from build123d import *

# Parameters (mm, degrees)
SKETCH_W        = 68
SKETCH_H        = 44
SKETCH_R        = 1.75
SKETCH_R_2      = 1.2
PAD_DEPTH       = 5
SKETCH001_R     = 3.6
SKETCH001_R_2   = 2.65
POCKET_DEPTH    = 2.5
SKETCH002_W     = 1.5
SKETCH002_H     = 4
PAD001_DEPTH    = 2
SKETCH003_R     = 0.9
POCKET001_DEPTH = 5
SKETCH004_W     = 16
SKETCH004_H     = 17
POCKET002_DEPTH = 1
SKETCH005_W     = 8
SKETCH005_H     = 3
PAD002_DEPTH    = 1
POCKET003_DEPTH = 27


with BuildPart() as part:
    # Sketch → Pad (new body)
    with BuildSketch(Plane.XY):
        Rectangle(SKETCH_W, SKETCH_H)
        with Locations((18, -16.75)):
            Circle(SKETCH_R, mode=Mode.SUBTRACT)
        with Locations((-18, -16.75)):
            Circle(SKETCH_R, mode=Mode.SUBTRACT)
        with Locations((-25, 14)):
            Circle(SKETCH_R_2, mode=Mode.SUBTRACT)
    extrude(amount=PAD_DEPTH)

    # Sketch001 (on Face9 of Pad) → Pocket (cut)
    with BuildSketch(Plane.XY.offset(5)):
        with Locations((-18, -16.75)):
            Circle(SKETCH001_R)
        with Locations((18, -16.75)):
            Circle(SKETCH001_R)
        with Locations((-25, 14)):
            Circle(SKETCH001_R_2)
    extrude(amount=-POCKET_DEPTH, mode=Mode.SUBTRACT)

    # Sketch002 (on Face5 of Pocket) → Pad001 (join)
    with BuildSketch(Plane.XY.offset(5)):
        Polygon((-16.5, -21), (16.5, -21), (16.5, -20.35), (18, -20.35), (18, -22), (-18, -22), (-18, -20.35), (-16.5, -20.35), align=None)
        Polygon((16.5, 15.4), (16.5, 13.4), (18, 13.4), (18, 22), (-18, 22), (-18, 13.4), (-16.5, 13.4), (-16.5, 15.4), align=None)
        with Locations((-17.25, -2.8)):
            Rectangle(SKETCH002_W, SKETCH002_H)
        with Locations((17.25, -2.8)):
            Rectangle(SKETCH002_W, SKETCH002_H)
    extrude(amount=PAD001_DEPTH)

    # Sketch003 (on Face34 of Pad001) → Pocket001 (cut)
    with BuildSketch(Plane.XY.offset(7)):
        with Locations((0, 16.5)):
            Circle(SKETCH003_R)
    extrude(amount=-POCKET001_DEPTH, mode=Mode.SUBTRACT)

    # Sketch004 (on Face5 of Pocket001) → Pocket002 (cut)
    with BuildSketch(Plane.XY.offset(5)):
        with Locations((26, 6.3)):
            Rectangle(SKETCH004_W, SKETCH004_H)
        with Locations((26, -11.9)):
            Rectangle(SKETCH004_W, SKETCH004_H)
        with Locations((-26, 6.3)):
            Rectangle(SKETCH004_W, SKETCH004_H)
        with Locations((-26, -11.9)):
            Rectangle(SKETCH004_W, SKETCH004_H)
    extrude(amount=-POCKET002_DEPTH, mode=Mode.SUBTRACT)

    # Sketch005 (on Face21 of Pocket002) → Pad002 (join, symmetric)
    with BuildSketch(Plane.XY.offset(7)):
        with Locations((-9.5, -20.5)):
            Rectangle(SKETCH005_W, SKETCH005_H)
        with Locations((9.5, -20.5)):
            Rectangle(SKETCH005_W, SKETCH005_H)
    extrude(amount=PAD002_DEPTH, both=True)

    # Sketch006 (on Face62 of Pad002) → Pocket003 (cut)
    with BuildSketch(Plane.YZ.offset(13.5)):
        Polygon((-19, 6), (-21, 6), (-19, 8), align=None)
    extrude(amount=-POCKET003_DEPTH, mode=Mode.SUBTRACT)


solid = part.part
Read the model definition and answer for the solid it produces. Units are mm, in the model's axes. A direction names the side the tool comes from. Round coordinates to 2 decimals unless told otherwise and drop trailing zeros. Write each loop counter-clockwise with the first axis right and the second up, starting at its lowest first coordinate (ties: lowest second). Pieces come first, ordered by that corner, then holes.
Q1. Find section A-A on x = -25. Determine the outline of the cut face in (y, z), and give its area (3 significant figures).
Values:
outline: (-22, 0) - (12.8, 0) - (12.8, 2.5) - (11.35, 2.5) - (11.35, 4) - (-2.2, 4) - (-2.2, 5) - (-3.4, 5) - (-3.4, 4) - (-20.4, 4) - (-20.4, 5) - (-22, 5) - close; (15.2, 0) - (22, 0) - (22, 5) - (16.65, 5) - (16.65, 2.5) - (15.2, 2.5) - close
area: 170 mm2
Q2. Flat-ended cylindrical pins translate along their axes: P1, Ø0.6, axis at y = -2, z = 6, coming from the +X side; P2, Ø12, axis at x = 13.5, y = 17.5, coming from the +Z side; P3, Ø2, axis at x = -17.5, y = -15.5, coming from the +Z side. Find the tip coordinate at first contact, or state that the pin passes through.
Values:
P1: stops at x = 18
P2: stops at z = 7
P3: stops at z = 2.5
Q3. The mould has two halves that part along Y. Classify faces 4 (the face through (0, 22, 3)), 5 (the face through (26, -12, 4)), 6 (the face through (-26, -12, 4)), 7 (the face through (-16.2, -21.3, 7)): released by +Y, released by -Y, zero draft, split by the parting line, or undercut.
Values:
face 4: released by +Y
face 5: undercut
face 6: undercut
face 7: zero draft
Q4. Find section B-B on y = -16.75. Determine the outline of the cut face in (x, z).
Values:
outline: (-34, 0) - (-19.75, 0) - (-19.75, 2.5) - (-21.6, 2.5) - (-21.6, 4) - (-34, 4) - close; (-16.25, 0) - (16.25, 0) - (16.25, 2.5) - (14.4, 2.5) - (14.4, 5) - (-14.4, 5) - (-14.4, 2.5) - (-16.25, 2.5) - close; (19.75, 0) - (34, 0) - (34, 4) - (21.6, 4) - (21.6, 2.5) - (19.75, 2.5) - close
Q5. Find section D-D on y = -6.5. Determine the outline of the cut face in (x, z), and give its area (3 significant figures).
Values:
outline: (-34, 0) - (34, 0) - (34, 4) - (18, 4) - (18, 5) - (-18, 5) - (-18, 4) - (-34, 4) - close
area: 308 mm2
Q6. Find section C-C on x = -9. Determine the outline of the cut face in (y, z), and give its area (3 significant figures).
Values:
outline: (-22, 0) - (22, 0) - (22, 7) - (15.4, 7) - (15.4, 5) - (-21, 5) - (-21, 6) - (-19, 8) - (-22, 8) - close
area: 238 mm2
Q7. Straight lines are drawn through the part: line 1 (Y direction, x = 18, z = 3.95); line 2 (X direction, y = -14, z = 3.5); line 3 (Z direction, x = 21.5, y = 1.5). For each, find the intervals that lie inside material, in ascending order.
Values:
line 1: y = -22 to -20.35, -13.15 to 22
line 2: x = -34 to -20.32, -15.68 to 15.68, 20.32 to 34
line 3: z = 0 to 4
Q8. A tool of negligible diameter and unlimited length cuts with its end or side. For faces 1 (the face through (16.3, -21.3, 7)), 2 (the face through (0, 17, 2)), 3 (the face through (17, -4.8, 6)), from which of +Z, -Z, +X, -X, +Y, -Y can it reach the whole face along a straight path? Write none if from no direction.
Values:
face 1: +Z, +X, +Y, -Y
face 2: +Z
face 3: +Z, +X, -X
